Autodesk Inventor part; units mm, degrees
ref_plane "YZ Plane" through (0, 0, 0) normal (1, 0, 0) x (0, 1, 0)
ref_plane "XZ Plane" through (0, 0, 0) normal (0, 1, 0) x (-1, 0, 0)
ref_plane "XY Plane" through (0, 0, 0) normal (0, 0, 1) x (1, 0, 0)
sketch "Sketch1" plane through (0, 0, 0) normal (0, 0, 1) x (1, 0, 0)
  circle A0 centre (0, 0) radius 3.25
  dimension "d0" = 6.5
extrude "Roller Base" add sketch "Sketch1" along normal mid plane 2.9
sketch "Sketch2" plane through (0, 0, 0) normal (0, 0, 1) x (1, 0, 0)
  circle A0 centre (0, 0) radius 0.975
  dimension "d3" = 1.95
extrude "Roller Axis" cut sketch "Sketch2" along normal through all both and the other way through all
sketch "Sketch3" plane through (0, 0, 0) normal (0, 0, 1) x (1, 0, 0)
  circle A0 centre (0, 0) radius 0.975
  circle A1 centre (0, 0) radius 3.25
  circle A2 centre (0, 0) radius 2.25
  dimension "d6" = 4.5
extrude "Roller Bar Fit" cut sketch "Sketch3" along normal mid plane 2.2 contours A1
properties part number "Roller" material "Brass, Soft Yellow, Welded"
Can you work these out from the model? Positions are in its coordinate system, mm. Round coordinates to 2 decimals unless told otherwise and drop trailing zeros. Order: outer loops, then holes, each group sorted by start corner. A loop starts at its lowest first (then second) coordinate and runs counter-clockwise, first axis right, second up. Notation, with made-up numbers: (53.5, 8.25) -> (57.5, 8.25) arc R16 ccw to (57.5, 26.25) -> close; hole circle Ø4 at (-16.5, -22.5). An arc over 180 degrees is marked (long way). Write each question's results on one line, items separated by ' | '. Start each with the question number.
Item 1: If we section it at D-D, the plane x = -1.25: Write out the boundary of the cut face in (y, z).
Item 2: Please list where these lines run through material, in increasing order: L1, parallel to Y at x = 0, z = 0 (3 decimals); L2, parallel to Z at x = -1.75, y = 1.5; L3, parallel to X at y = -0.75, z = 0.
Item 3: If we section it at C-C, the plane z = 0.85: Write out the boundary of the cut face in (x, y) (3 decimals).
Item 4: Thinking about a two-plate mould opening in Z: for faces 1 (the flat face through (1, 1, 1.45)), 2 (the cylindrical face through (-2.579, -1.978, -1.273)), 3 (the cylindrical face through (-0.29, -2.23, -0.02)), which applies, +Z half, -Z half, draft (parallel to the pull), parting line (faces both ways), or undercut?
Item 5: If we section it at A-A, the plane y = 0: Write out the boundary of the cut face in (x, z) (3 decimals), then the cut area to 4 significant figures.
Results:
1) outline: (-3, -1.45) -> (3, -1.45) -> (3, -1.1) -> (1.87, -1.1) -> (1.87, 1.1) -> (3, 1.1) -> (3, 1.45) -> (-3, 1.45) -> (-3, 1.1) -> (-1.87, 1.1) -> (-1.87, -1.1) -> (-3, -1.1) -> close
2) L1: y = -2.25 to -0.975, 0.975 to 2.25 | L2: z = -1.45 to -1.1, 1.1 to 1.45 | L3: x = -2.12 to -0.62, 0.62 to 2.12
3) outline: circle Ø4.5 at (0, 0); hole circle Ø1.95 at (0, 0)
4) face 1: +Z half | face 2: draft | face 3: undercut
5) outline: (-3.25, -1.45) -> (-0.975, -1.45) -> (-0.975, 1.45) -> (-3.25, 1.45) -> (-3.25, 1.1) -> (-2.25, 1.1) -> (-2.25, -1.1) -> (-3.25, -1.1) -> close; (0.975, -1.45) -> (3.25, -1.45) -> (3.25, -1.1) -> (2.25, -1.1) -> (2.25, 1.1) -> (3.25, 1.1) -> (3.25, 1.45) -> (0.975, 1.45) -> close | area: 8.795 mm2
